from build123d import *

# Parameters (mm, degrees)
SKETCH1_R           = 11
SKETCH1_R_2         = 1.5
BOSS_EXTRUDE1_DEPTH = 2
SKETCH2_R           = 4.5
SKETCH2_R_2         = 2.5
BOSS_EXTRUDE2_DEPTH = 3
SKETCH3_R           = 0.5
CUT_EXTRUDE1_DEPTH  = 16.842979518
CIRPATTERN1_COUNT   = 4


with BuildPart() as part:
    # Sketch1 → Boss-Extrude1 (new body)
    with BuildSketch(Plane(origin=(0, 0, 0), x_dir=(1, 0, 0), z_dir=(0, 1, 0))):
        with Locations(Location((0, 0, 0), (0, 0, 270))):
            Circle(SKETCH1_R)
        with Locations(Location((0, 0, 0), (0, 0, 270))):
            Circle(SKETCH1_R_2, mode=Mode.SUBTRACT)
    extrude(amount=BOSS_EXTRUDE1_DEPTH)

    # Sketch2 → Boss-Extrude2 (add)
    with BuildSketch(Plane(origin=(0, 2, 0), x_dir=(1, 0, 0), z_dir=(0, 1, 0))):
        with Locations(Location((0, 0, 0), (0, 0, 270))):
            Circle(SKETCH2_R)
        with Locations(Location((0, 0, 0), (0, 0, 270))):
            Circle(SKETCH2_R_2, mode=Mode.SUBTRACT)
    extrude(amount=BOSS_EXTRUDE2_DEPTH)

    # Sketch3 → Cut-Extrude1 (cut, through all)
    with BuildSketch(Plane(origin=(0, 2, 0), x_dir=(1, 0, 0), z_dir=(0, 1, 0))):
        with Locations(Location((-3.5, 7.25, 0), (0, 0, 270))):
            Circle(SKETCH3_R)
        with Locations(Location((0, 7.25, 0), (0, 0, 270))):
            Circle(SKETCH3_R)
        with Locations(Location((3.5, 7.25, 0), (0, 0, 270))):
            Circle(SKETCH3_R)
    cut_extrude1 = extrude(amount=-CUT_EXTRUDE1_DEPTH, mode=Mode.SUBTRACT)

    # CirPattern1: Cut-Extrude1 ×4 about axis
    cirpattern1_axis = Axis((0, 0, 0), (0, 1, 0))
    for i in range(1, CIRPATTERN1_COUNT):
        add(cut_extrude1.rotate(cirpattern1_axis, i * 360 / CIRPATTERN1_COUNT), mode=Mode.SUBTRACT)


solid = part.part
Source: CAD feature listing. Evaluate the final solid. Frame: model axes, mm. A direction names the side the tool comes from. Round coordinates to 2 decimals unless told otherwise and drop trailing zeros. Loops run counter-clockwise (first coordinate to the right, second up) from the corner with the lowest first, then second, coordinate; pieces in that order, holes last. Notation, with made-up numbers: M 1.5,-31 L 59.5,-31 A9 cw 59.5,-25 Z; hole C 47,-25.75 d6. An arc over 180 degrees is marked long. Return JSON: item names as keys, results as strings. Group by question number.
1. Section query C-C on z = 7.25. Output: boundary loops of the cut face in (x, y).
2. Reachability of faces 4 (the face through (-2.44, 3.48, -0.54)), 5 (the face through (3.65, 1.014, -6.773)) from +Z, -Z, +X, -X, +Y, -Y: full face, straight path, thin tool, end or side. Return the list, or none.
3. Pin query (flat end, axial travel): pin 1 (2 mm diameter, centred on x = -8.5, z = 5.5, fed in from +Y); pin 2 (1 mm diameter, centred on x = 2, y = 4, fed in from +Z); pin 3 (1.5 mm diameter, centred on y = 1.5, z = 7.5, fed in from +X). Return the tip coordinate at first contact, or that it passes through.
4. Section query D-D on z = 1. Output: boundary loops of the cut face in (x, y), and give its area (3 significant figures).
5. Section query B-B on x = 3.5. Output: boundary loops of the cut face in (y, z).
6. Section query A-A on y = 0.75. State how many separate pieces and enclosed holes the cut face has, and give its area (3 significant figures).
7. Material intervals for line 1 along X through (y, z) = (0.6, -7.25); line 2 along Y through (x, z) = (5.25, -2.25); line 3 along Z through (x, y) = (-1.75, 4.7), sorted ascending. Write a range as from..to.
8. Mould query, pull axis X, two halves, no side actions, for faces 1 (the face through (-2, 5, 2)), 2 (the face through (1.352, 3.479, 4.292)), 3 (the face through (6.773, 1.014, -3.35)). Classes: released by +X, released by -X, zero draft, split by the parting line, or undercut.
Checks:
{
 "1": {"outline": "M -8.27,0 L -4,0 L -4,2 L -8.27,2 Z; M -3,0 L -0.5,0 L -0.5,2 L -3,2 Z; M 0.5,0 L 3,0 L 3,2 L 0.5,2 Z; M 4,0 L 8.27,0 L 8.27,2 L 4,2 Z"},
 "2": {"face 4": "+Y", "face 5": "+Y, -Y"},
 "3": {"pin 1": "stops at y = 2", "pin 2": "stops at z = 4.24", "pin 3": "stops at x = 8.69"},
 "4": {"outline": "M -10.95,0 L -1.12,0 L -1.12,2 L -2.29,2 L -2.29,5 L -4.39,5 L -4.39,2 L -10.95,2 Z; M 1.12,0 L 10.95,0 L 10.95,2 L 4.39,2 L 4.39,5 L 2.29,5 L 2.29,2 L 1.12,2 Z", "area": "51.9 mm²"},
 "5": {"outline": "M 0,-10.43 L 2,-10.43 L 2,-7.75 L 0,-7.75 Z; M 0,-6.75 L 2,-6.75 L 2,-2.83 L 5,-2.83 L 5,2.83 L 2,2.83 L 2,6.75 L 0,6.75 Z; M 0,7.75 L 2,7.75 L 2,10.43 L 0,10.43 Z"},
 "6": {"separate pieces": "1", "enclosed holes": "13", "area": "364 mm²"},
 "7": {"line 1": "x = -8.27..-4, -3..-0.5, 0.5..3, 4..8.27", "line 2": "y = 0..2", "line 3": "z = -4.15..-1.79, 1.79..4.15"},
 "8": {"face 1": "zero draft", "face 2": "split by the parting line", "face 3": "undercut"}
}
